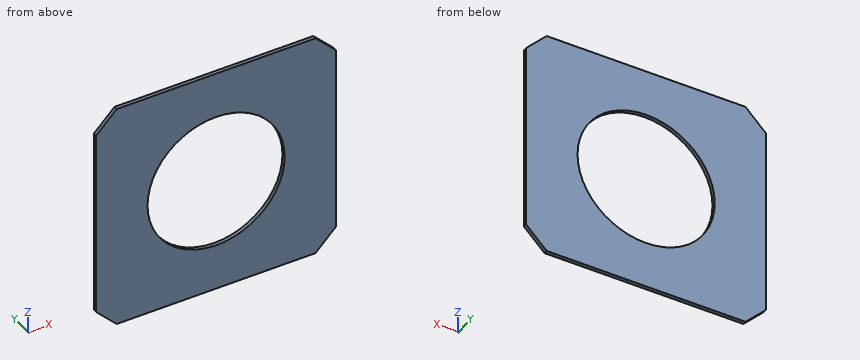
from build123d import *

# Parameters (mm, degrees)
F0_W     = 222.25
F0_H     = 212.725
F0_R     = 63.5
F1_DEPTH = 3.429
F2_SIZE  = 19.05


with BuildPart() as f1:
    # F0 (on Front) → F1 (new body)
    with BuildSketch(Plane.XZ):
        Rectangle(F0_W, F0_H)
        Circle(F0_R, mode=Mode.SUBTRACT)
    extrude(amount=F1_DEPTH)

    # F2
    f2_edges = [f1.edges().sort_by_distance(p)[0] for p in [
        (-111.125, -1.7145, 106.3625),
        (111.125, -1.7145, 106.3625),
        (-111.125, -1.7145, -106.3625),
        (111.125, -1.7145, -106.3625),
    ]]
    chamfer(f2_edges, length=F2_SIZE)


solid = f1.part
CAD build for the part. Positions are in the model's coordinates, mm. Coordinates: 2 decimals unless noted, no trailing zeros. Write each loop counter-clockwise with the first axis right and the second up, starting at its lowest first coordinate (ties: lowest second). Pieces come first, ordered by that corner, then holes. Notation, with made-up numbers: M 56,62.5 L 95,62.5 A17 cw 95,67.5 Z; hole C -30.75,18 d9. An arc over 180 degrees is marked long. Answer as a JSON object with one key per item and string values. Group by question number.
1) Saw through at B-B (y = -1.8). Write the cut outline in (x, z) (1 decimal).
2) Saw through at D-D (z = -92.5). Write the cut outline in (x, y).
3) Wall check: line 1 (Z direction, x = 7.5, y = -0.85); line 2 (X direction, y = -2.9, z = -23) (3 decimals); line 3 (Z direction, x = -16.5, y = -2.2). Give the ranges that are in metal, low to high. Write a range as from..to.
4) Saw through at A-A (x = 0). Write the cut outline in (y, z).
5) Saw through at C-C (z = 0). Write the cut outline in (x, y) (3 decimals), plus the area to 3 significant figures.
Values follow:
{
 "1": {"outline": "M -111.1,-87.3 L -92.1,-106.4 L 92.1,-106.4 L 111.1,-87.3 L 111.1,87.3 L 92.1,106.4 L -92.1,106.4 L -111.1,87.3 Z; hole C 0,0 d127"},
 "2": {"outline": "M -105.94,-3.43 L 105.94,-3.43 L 105.94,0 L -105.94,0 Z"},
 "3": {"line 1": "z = -106.36..-63.06, 63.06..106.36", "line 2": "x = -111.125..-59.188, 59.188..111.125", "line 3": "z = -106.36..-61.32, 61.32..106.36"},
 "4": {"outline": "M -3.43,-106.36 L 0,-106.36 L 0,-63.5 L -3.43,-63.5 Z; M -3.43,63.5 L 0,63.5 L 0,106.36 L -3.43,106.36 Z"},
 "5": {"outline": "M -111.125,-3.429 L -63.5,-3.429 L -63.5,0 L -111.125,0 Z; M 63.5,-3.429 L 111.125,-3.429 L 111.125,0 L 63.5,0 Z", "area": "327 mm2"}
}
